Part model, mm, in its own coordinate system. A direction names the side the tool comes from. Round coordinates to 2 decimals unless told otherwise and drop trailing zeros. Write each loop counter-clockwise with the first axis right and the second up, starting at its lowest first coordinate (ties: lowest second). Pieces come first, ordered by that corner, then holes. Notation, with made-up numbers: (-8.5, 88) -> (48.5, 88) arc R27 cw to (48.5, 108) -> close; hole circle Ø4 at (46.5, 6.5). An arc over 180 degrees is marked (long way). Use CSV: the item, a comma, the result in double quotes. Start each with the question number.
```python
from build123d import *

# Parameters (mm, degrees)
SKETCH1_W           = 21
SKETCH1_H           = 21
SKETCH1_R           = 3.5
BOSS_EXTRUDE1_DEPTH = 4
BOSS_EXTRUDE2_DEPTH = 4
SKETCH3_W           = 2.85
SKETCH3_H           = 2.205413133
CUT_EXTRUDE1_DEPTH  = 4


with BuildPart() as part:
    # Sketch1 → Boss-Extrude1 (new body)
    with BuildSketch(Plane.XY):
        Rectangle(SKETCH1_W, SKETCH1_H)
        Circle(SKETCH1_R, mode=Mode.SUBTRACT)
    extrude(amount=BOSS_EXTRUDE1_DEPTH)

    # Sketch2 → Boss-Extrude2 (add)
    with BuildSketch(Plane(origin=(0, 0, 0), x_dir=(-1, 0, 0), z_dir=(0, 0, -1))):
        with BuildLine():
            Line((0, 10.5), (0, 9))
            ThreePointArc((0, 9), (-9, 0), (0, -9))
            Line((0, -9), (0, -10.5))
            ThreePointArc((0, -10.5), (-10.5, 0), (0, 10.5))
        make_face()
    extrude(amount=BOSS_EXTRUDE2_DEPTH)

    # Sketch3 → Cut-Extrude1 (cut)
    with BuildSketch(Plane(origin=(0, 0, 0), x_dir=(-1, 0, 0), z_dir=(0, 0, -1))):
        with Locations((0, 8.361109671)):
            Rectangle(SKETCH3_W, SKETCH3_H)
    extrude(amount=-CUT_EXTRUDE1_DEPTH, mode=Mode.SUBTRACT)


solid = part.part
```
1. Flat gauge pins, fed straight in: pin 1 (1.2 mm diameter, centred on y = 9.5, z = -2, fed in from -X); pin 2 (5.5 mm diameter, centred on x = 0, y = 0, fed in from -Z); pin 3 (1 mm diameter, centred on x = 5.5, z = -2, fed in from +Y). Where does each tip first touch, or does it go through?
2. Band-saw the part on A-A (x = -3). List the corners of the cut face in (y, z).
3. Drill centre lines: line 1 along Y through (x, z) = (0, 2.5); line 2 along Y through (x, z) = (1, 2.75); line 3 along X through (y, z) = (8.25, 1.5) (3 decimals). Where is each one in solid material? Low to high. Write a range as [from, to].
4. Band-saw the part on C-C (y = 2.25). List the corners of the cut face in (x, z), then the cut area to 3 significant figures.
5. Band-saw the part on D-D (y = -5). List the corners of the cut face in (x, z), then the cut area to 3 significant figures.
6. Which spindle directions (+Z, -Z, +X, -X, +Y, -Y) get a long thin tool onto all of the face, cutting with end or side? Do faces 1 (the flat face through (-1.425, 8, 2)), 2 (the flat face through (0, -10, -2)), 3 (the flat face through (8, 8, 0)), 4 (the flat face through (1.425, 8, 2)), 5 (the cylindrical face through (9, 0, -2)). Say none if no direction does.
7. Band-saw the part on B-B (z = 0.5). List the corners of the cut face in (x, y) (3 decimals).
Answers below:
1,pin 1,"stops at x = 0"
1,pin 2,"passes through"
1,pin 3,"stops at y = 9.23"
2,outline,"(-10.5, 0) -> (-1.8, 0) -> (-1.8, 4) -> (-10.5, 4) -> close; (1.8, 0) -> (10.5, 0) -> (10.5, 4) -> (1.8, 4) -> close"
3,line 1,"y = [-10.5, -3.5], [3.5, 7.26], [9.46, 10.5]"
3,line 2,"y = [-10.5, -3.35], [3.35, 7.26], [9.46, 10.5]"
3,line 3,"x = [-10.5, -1.425], [1.425, 10.5]"
4,outline,"(-10.5, 0) -> (-2.68, 0) -> (-2.68, 4) -> (-10.5, 4) -> close; (2.68, 0) -> (8.71, 0) -> (8.71, -4) -> (10.26, -4) -> (10.26, 0) -> (10.5, 0) -> (10.5, 4) -> (2.68, 4) -> close"
4,area,"68.7 mm^2"
5,outline,"(-10.5, 0) -> (7.48, 0) -> (7.48, -4) -> (9.23, -4) -> (9.23, 0) -> (10.5, 0) -> (10.5, 4) -> (-10.5, 4) -> close"
5,area,"91.0 mm^2"
6,face 1,"+Z, -Z"
6,face 2,"-Z, -X, +Y, -Y"
6,face 3,"-Z, +X, +Y"
6,face 4,"+Z"
6,face 5,"-Z, -X"
7,outline,"(-10.5, -10.5) -> (10.5, -10.5) -> (10.5, 10.5) -> (-10.5, 10.5) -> close; hole circle Ø7 at (0, 0); hole (-1.425, 7.258) -> (1.425, 7.258) -> (1.425, 9.464) -> (-1.425, 9.464) -> close"
